Part model, mm, in its own coordinate system. A direction names the side the tool comes from. Coordinates: 2 decimals unless noted, no trailing zeros. Loops run counter-clockwise (first coordinate to the right, second up) from the corner with the lowest first, then second, coordinate; pieces in that order, holes last. Notation, with made-up numbers: (65, 61.25) - (97, 61.25) arc R31 ccw to (97, 88.25) - close; hole circle Ø10 at (71, 80). An arc over 180 degrees is marked (long way). Answer as CSV lines item,"result".
Autodesk Fusion 360 part; units mm, degrees
sketch "arm sketch" plane through (0, 0, 0) normal (0, 0, 1) x (1, 0, 0)
  circle A0 centre (-0.0034, 0.0021) radius 3.65
  arc A1 (-0.0006, -3.625) -> (0, -3.625) centre (0, 0) ccw
  line L0 (0, -3.625) -> (0, -3.6479)
  line L1 (0, -3.625) -> (0, -3.6479)
  line L2 (1.986, 14.5075) -> (3.33, 1.4889)
  line L3 (-3.3369, 1.4889) -> (-2.0034, 14.2947)
  line L4 (-3.3369, -1.4847) -> (-1.9929, -14.5033)
  line L5 (1.9965, -14.3152) -> (3.3333, -1.4773)
  line L6 (-4.0034, 16.3021) -> (-5.0034, 0.0021)
  line L7 (3.9966, 16.3021) -> (4.9966, 0.0021)
  line L8 (4.9966, 0.0021) -> (4.9966, -16.9979)
  line L9 (-5.0034, -17.9979) -> (-5.0034, 0.0021)
  line L10 (4.9966, -16.9979) -> (-5.0034, -16.9979)
  line L11 (-0.0449, 98) -> (7.9551, 98.0037)
  line L12 (-0.0449, 98) -> (-8.0449, 97.9963)
  line L13 (-4.0034, 16.3021) -> (-4.0449, 97.9982)
  line L14 (3.9966, 16.3021) -> (3.9551, 98.0018)
  line L15 (-8.0449, 97.9963) -> (-8.0458, 99.9963)
  line L16 (-8.0458, 99.9963) -> (7.9542, 100.0044)
  line L17 (7.9542, 100.0044) -> (7.9551, 98.0037)
  arc A2 (-1.9929, -14.5033) -> (1.9965, -14.3152) centre (-0.0034, -14.2979) ccw
  arc A3 (1.986, 14.5075) -> (-2.0034, 14.2947) centre (-0.0034, 14.3021) ccw
  dimension "d13" = 7.3
  dimension "d30" = 14.3
  dimension "d31" = 14.3
  dimension "d32" = 4
  dimension "d33" = 4
  dimension "d50" = 5
  dimension "d52" = 5
  dimension "d55" = 1
  dimension "d69" = 98
  dimension "d71" = 8
  dimension "d72" = 8
  dimension "d73" = 2
  dimension "d74" = 16
extrude "Extrude14" add sketch "arm sketch" along normal blind 2.5 contours A0 L2 L3 A3 | A0 L4 L5 A2 makes body 1 at (-0.0069, 10.8181, 0) makes body 2 at (0.0014, -10.8221, 0)
extrude "Extrude15" add sketch "arm sketch" along normal blind 5 contours L6 L7 L8 L9 L10 L11 L12 L13 L14 bodies 1 2
extrude "Extrude16" add sketch "arm sketch" along normal blind 13 contours L11 L12 L15 L16 L17 bodies 1
sketch "bolts" plane through (-0.0507, 100.0004, 0) normal (-0.0005, 1, 0) x (-1, -0.0005, 0)
  line L0 (-8.0049, 0) -> (7.9951, 0)
  line L1 (7.9951, 0) -> (7.9951, 13)
  line L2 (7.9951, 13) -> (-8.0049, 13)
  line L3 (-8.0049, 13) -> (-8.0049, 0)
  circle A0 centre (-4.0049, 9) radius 2
  circle A1 centre (3.9951, 9) radius 2
  dimension "d85" = 8
  dimension "d86" = 4
  dimension "d87" = 4
extrude "Extrude17" cut sketch "bolts" against normal blind 5 contours A0 | A1 bodies 1
Q1. Flat gauge pins, fed straight in: pin 1 (3 mm diameter, centred on x = -2.5, y = 44, fed in from +Z); pin 2 (5.5 mm diameter, centred on y = -5.5, z = 1.5, fed in from -X); pin 3 (1.5 mm diameter, centred on y = -5.5, z = 2, fed in from +X). Where does each tip first touch, or does it go through?
Results:
pin 1,"stops at z = 5"
pin 2,"stops at x = -5"
pin 3,"stops at x = 5"
Q2. Saw through at B-B (y = 87.5). Give the cut face in (x, z), then the cut area to 3 significant figures.
Results:
outline,"(-4.04, 0) - (3.96, 0) - (3.96, 5) - (-4.04, 5) - close"
area,"40.0 mm^2"
Q3. Wall check: L1, parallel to X at y = 46.5, z = 4; L2, parallel to Y at x = -6, z = 4.5; L3, parallel to Z at x = 2.25, y = 71. Give the ranges that are in metal, low to high.
Results:
L1,"x = -4.02 to 3.98"
L2,"y = 98 to 100"
L3,"z = 0 to 5"
Q4. Saw through at A-A (y = 2.5). Give the cut face in (x, z).
Results:
outline,"(-4.85, 0) - (-2.66, 0) - (-2.66, 2.5) - (-3.23, 2.5) - (-3.23, 5) - (-4.85, 5) - close; (2.66, 0) - (4.84, 0) - (4.84, 5) - (3.23, 5) - (3.23, 2.5) - (2.66, 2.5) - close"
Q5. Two-plate mould, pull along Y, no slides. Class faces 1 (the face through (0, -16.998, 2)), 2 (the face through (0, 42, 0)), 3 (the face through (0.133, -16.293, 3.732)): released by +Y, released by -Y, zero draft, split by the parting line, or undercut.
Results:
face 1,"released by -Y"
face 2,"zero draft"
face 3,"undercut"
Q6. Which spindle directions (+Z, -Z, +X, -X, +Y, -Y) get a long thin tool onto all of the face, cutting with end or side? Do faces 4 (the face through (-5.003, -9, 2)), 5 (the face through (2.656, -7.986, 3.732)), 6 (the face through (4.997, -8, 2)). Say none if no direction does.
Results:
face 4,"+Z, -Z, -X, -Y"
face 5,"+Z"
face 6,"+Z, -Z, +X, -Y"
